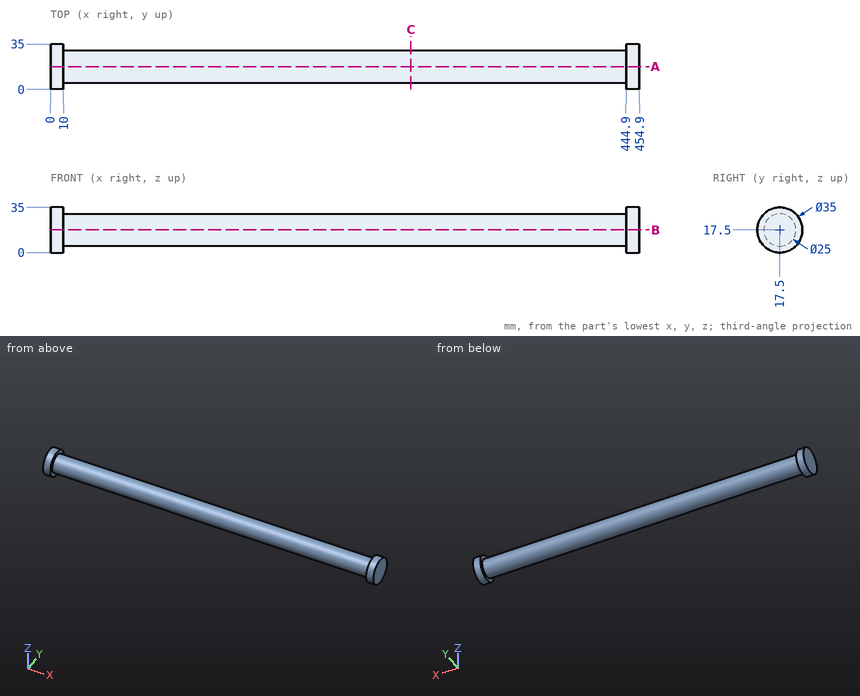
Could you check a few things on this drawing? It's one solid part, dimensions in mm from its lowest x, y, z. Give positions to 0.01 mm unless a question says otherwise; leave off trailing zeros. Write each loop counter-clockwise with the first axis right and the second up, starting at its lowest first coordinate (ties: lowest second). Pieces come first, ordered by that corner, then holes.
(1) If I drill on L1, parallel to X at y = 9, z = 27; L2, parallel to Z at x = 26, y = 16; L3, parallel to Y at x = 54, z = 18, over which ranges is the centre line in solid material (lowest first)?
Output values:
L1: x = 0 to 10, 444.9 to 454.9
L2: z = 5.09 to 29.91
L3: y = 5.01 to 29.99
(2) Will these pins go through, and if not, where does the flat tip stop? pin 1 (8 mm diameter, centred on x = 378.5, z = 24.5, fed in from -Y); pin 2 (10 mm diameter, centred on x = 54, y = 22.5, fed in from -Z); pin 3 (3 mm diameter, centred on x = 169.5, y = 27, fed in from +Z).
Output values:
pin 1: stops at y = 5.37
pin 2: stops at z = 5
pin 3: stops at z = 27.1
(3) Imagine slicing it at A-A, the plane y = 17.5. Write out the boundary of the cut face in (x, z).
Output values:
outline: (0, 0) - (10, 0) - (10, 5) - (444.9, 5) - (444.9, 0) - (454.9, 0) - (454.9, 35) - (444.9, 35) - (444.9, 30) - (10, 30) - (10, 35) - (0, 35) - close
(4) Imagine slicing it at C-C, the plane x = 278.5. Write out the boundary of the cut face in (y, z).
Output values:
outline: circle Ø25 at (17.5, 17.5)
